```python
from build123d import *
from build123d.topology import SkipClean

# Parameters (mm, degrees)
ESQUISSE1_W             = 300
ESQUISSE1_H             = 280
BOSS_EXTRU_1_DEPTH      = 4
ESQUISSE2_W             = 80
ESQUISSE2_H             = 120
ENL_V_MAT_EXTRU_1_DEPTH = 206.221831197
ESQUISSE4_W             = 67
ESQUISSE4_H             = 60
ENL_V_MAT_EXTRU_3_DEPTH = 206.221831197
BOSS_EXTRU_2_DEPTH      = 4
ESQUISSE6_R             = 2.1
ENL_V_MAT_EXTRU_4_DEPTH = 211.059515376
BOSS_EXTRU_3_DEPTH      = 4
BOSS_EXTRU_4_DEPTH      = 4
ESQUISSE9_R             = 2.1
ENL_V_MAT_EXTRU_5_DEPTH = 244.522565689
ESQUISSE10_R            = 2.1
ENL_V_MAT_EXTRU_6_DEPTH = 244.522565689
ESQUISSE11_R            = 2.1
ENL_V_MAT_EXTRU_7_DEPTH = 244.522565689
BOSS_EXTRU_5_START      = -4
ESQUISSE12_R            = 5
ESQUISSE12_R_2          = 2.1
BOSS_EXTRU_5_DEPTH      = 4


with BuildPart() as part:
    # Esquisse1 → Boss.-Extru.1 (new body)
    with BuildSketch(Plane.XY):
        Rectangle(ESQUISSE1_W, ESQUISSE1_H)
    extrude(amount=BOSS_EXTRU_1_DEPTH)

    # Esquisse2 → Enl_v. mat.-Extru.1 (cut, through all)
    with BuildSketch(Plane.XY.offset(4)):
        with Locations((77.5, -80)):
            Rectangle(ESQUISSE2_W, ESQUISSE2_H)
        with Locations((-77.5, -80)):
            Rectangle(ESQUISSE2_W, ESQUISSE2_H)
    extrude(amount=-ENL_V_MAT_EXTRU_1_DEPTH, mode=Mode.SUBTRACT)

    # Esquisse4 → Enl_v. mat.-Extru.3 (cut, through all)
    with BuildSketch(Plane(origin=(0, 0, 0), x_dir=(-1, 0, 0), z_dir=(0, 0, -1))):
        with Locations((0, 110)):
            Rectangle(ESQUISSE4_W, ESQUISSE4_H)
    extrude(amount=-ENL_V_MAT_EXTRU_3_DEPTH, mode=Mode.SUBTRACT)

    # Esquisse5 → Boss.-Extru.2 (add)
    with BuildSketch(Plane(origin=(0, 0, 0), x_dir=(-1, 0, 0), z_dir=(0, 0, -1))):
        with BuildLine():
            Line((-128.75, -142), (-128.75, -140))
            Line((-128.75, -140), (-138.75, -140))
            Line((-138.75, -140), (-138.75, -142))
            ThreePointArc((-138.75, -142), (-133.75, -147), (-128.75, -142))
        make_face()
        with BuildLine():
            Line((138.75, -140), (128.75, -140))
            Line((128.75, -140), (128.75, -142))
            ThreePointArc((128.75, -142), (133.75, -147), (138.75, -142))
            Line((138.75, -142), (138.75, -140))
        make_face()
    extrude(amount=-BOSS_EXTRU_2_DEPTH)

    # Esquisse6 → Enl_v. mat.-Extru.4 (cut, through all)
    with BuildSketch(Plane(origin=(0, 0, 0), x_dir=(-1, 0, 0), z_dir=(0, 0, -1))):
        with Locations((-133.75, -142)):
            Circle(ESQUISSE6_R)
        with Locations((133.75, -142)):
            Circle(ESQUISSE6_R)
    extrude(amount=-ENL_V_MAT_EXTRU_4_DEPTH, mode=Mode.SUBTRACT)

    # Esquisse7 → Boss.-Extru.3 (add)
    with BuildSketch(Plane(origin=(0, 0, 0), x_dir=(-1, 0, 0), z_dir=(0, 0, -1))):
        Polygon((-150, 140), (-150, 184.8), (150, 184.8), (150, 140), (80, 140), (80, 145.2), (-80, 145.2), (-80, 140), align=None)
    extrude(amount=-BOSS_EXTRU_3_DEPTH)

    # Esquisse8 → Boss.-Extru.4 (add)
    with BuildSketch(Plane(origin=(0, 0, 0), x_dir=(-1, 0, 0), z_dir=(0, 0, -1))):
        with BuildLine():
            Line((-150, 184.8), (-150, 188.8))
            Line((-150, 188.8), (-114.582575695, 188.8))
            ThreePointArc((-114.582575695, 188.8), (-110, 191.8), (-105.417424305, 188.8))
            Line((-105.417424305, 188.8), (-70, 188.8))
            Line((-70, 188.8), (-70, 184.8))
            Line((-70, 184.8), (-150, 184.8))
        make_face()
        with BuildLine():
            Line((105.417424305, 188.8), (70, 188.8))
            Line((70, 188.8), (70, 184.8))
            Line((70, 184.8), (150, 184.8))
            Line((150, 184.8), (150, 188.8))
            Line((150, 188.8), (114.582575695, 188.8))
            ThreePointArc((114.582575695, 188.8), (110, 191.8), (105.417424305, 188.8))
        make_face()
    extrude(amount=-BOSS_EXTRU_4_DEPTH)

    # Esquisse9 → Enl_v. mat.-Extru.5 (cut, through all)
    with BuildSketch(Plane(origin=(0, 0, 0), x_dir=(-1, 0, 0), z_dir=(0, 0, -1))):
        with Locations((-110, 186.8)):
            Circle(ESQUISSE9_R)
        with Locations((110, 186.8)):
            Circle(ESQUISSE9_R)
    extrude(amount=-ENL_V_MAT_EXTRU_5_DEPTH, mode=Mode.SUBTRACT)

    # Esquisse10 → Enl_v. mat.-Extru.6 (cut, through all)
    with BuildSketch(Plane(origin=(0, 0, 0), x_dir=(-1, 0, 0), z_dir=(0, 0, -1))):
        with Locations((115, 142.5)):
            Circle(ESQUISSE10_R)
        with Locations(Location((-115, 142.5, 0), (0, 0, 180))):
            Circle(ESQUISSE10_R)
    extrude(amount=-ENL_V_MAT_EXTRU_6_DEPTH, mode=Mode.SUBTRACT)

    # Esquisse11 → Enl_v. mat.-Extru.7 (cut, through all)
    with BuildSketch(Plane.XY.offset(4)):
        with Locations((35.5, 110)):
            Circle(ESQUISSE11_R)
        with Locations((119.5, 110)):
            Circle(ESQUISSE11_R)
        with Locations(Location((-119.5, 110, 0), (0, 0, 180))):
            Circle(ESQUISSE11_R)
        with Locations((-35.5, 110)):
            Circle(ESQUISSE11_R)
    extrude(amount=-ENL_V_MAT_EXTRU_7_DEPTH, mode=Mode.SUBTRACT)

    # Esquisse12 → Boss.-Extru.5 (add)
    # profile 1 of 2: a face of its own
    with SkipClean():  # the faces are left unmerged after this step: merging them gives an invalid solid
        with BuildSketch(Plane(origin=(0, 0, 0), x_dir=(-1, 0, 0), z_dir=(0, 0, -1)).offset(BOSS_EXTRU_5_START)):
            with Locations((-35.5, 110)):
                Circle(ESQUISSE12_R)
            with Locations(Location((-35.5, 110, 0), (0, 0, 180))):
                Circle(ESQUISSE12_R_2, mode=Mode.SUBTRACT)
        # profile 2 of 2: a face of its own
        with BuildSketch(Plane(origin=(0, 0, 0), x_dir=(-1, 0, 0), z_dir=(0, 0, -1)).offset(BOSS_EXTRU_5_START)):
            with Locations((35.5, 110)):
                Circle(ESQUISSE12_R)
            with Locations((35.5, 110)):
                Circle(ESQUISSE12_R_2, mode=Mode.SUBTRACT)
        extrude(amount=BOSS_EXTRU_5_DEPTH)
    add(part.part.scale(1), mode=Mode.REPLACE)  # the faces are merged on a copy


solid = part.part
```
CAD build for the part. Positions are in the model's coordinates, mm. Coordinates: 2 decimals unless noted, no trailing zeros. Write each loop counter-clockwise with the first axis right and the second up, starting at its lowest first coordinate (ties: lowest second). Pieces come first, ordered by that corner, then holes. Notation, with made-up numbers: (-30, -26) -> (-8, -26) arc R4 cw to (-8, -22) -> close; hole circle Ø6 at (-9.5, -17). An arc over 180 degrees is marked (long way). Return JSON: item names as keys, results as strings. Group by question number.
Q1. Cut at B-B, the plane y = -61. Give the cut face in (x, z).
Q2. Cut at C-C, the plane x = -52.5. Give the cut face in (y, z), then the cut area to 3 significant figures.
Q3. Cut at D-D, the plane z = 2.7. State how many separate pieces and enclosed holes the cut face has, then the cut area to 3 significant figures.
Q4. Cut at A-A, the plane x = 2. Give the cut face in (y, z), then the cut area to 3 significant figures.
Q5. Flat gauge pins, fed straight in: pin 1 (2 mm diameter, centred on y = -141.5, z = 1.5, fed in from -X); pin 2 (2 mm diameter, centred on x = 144.5, z = 1.5, fed in from -Y); pin 3 (2 mm diameter, centred on x = 83.5, z = 2.5, fed in from +Y). Where does each tip first touch, or does it go through?
Q6. Drill centre lines: line 1 (X direction, y = -111, z = 3.2); line 2 (X direction, y = 186.8, z = 3.1); line 3 (Y direction, x = -61, z = 1.4). Where is each one in solid material? Low to high.
Returned:
{
 "1": {"outline": "(-150, 0) -> (-117.5, 0) -> (-117.5, 4) -> (-150, 4) -> close; (-37.5, 0) -> (37.5, 0) -> (37.5, 4) -> (-37.5, 4) -> close; (117.5, 0) -> (150, 0) -> (150, 4) -> (117.5, 4) -> close"},
 "2": {"outline": "(-20, 0) -> (140, 0) -> (140, 4) -> (-20, 4) -> close; (145.2, 0) -> (184.8, 0) -> (184.8, 4) -> (145.2, 4) -> close", "area": "798 mm2"},
 "3": {"separate pieces": "1", "enclosed holes": "11", "area": "74,100 mm2"},
 "4": {"outline": "(-140, 0) -> (80, 0) -> (80, 4) -> (-140, 4) -> close; (145.2, 0) -> (184.8, 0) -> (184.8, 4) -> (145.2, 4) -> close", "area": "1,040 mm2"},
 "5": {"pin 1": "stops at x = -138.75", "pin 2": "stops at y = -140", "pin 3": "stops at y = 188.8"},
 "6": {"line 1": "x = -150 to -117.5, -37.5 to 37.5, 117.5 to 150", "line 2": "x = -150 to -112.1, -107.9 to -70, 70 to 107.9, 112.1 to 150", "line 3": "y = -20 to 140, 145.2 to 184.8"}
}
